For this review, take the finished solid that the model builds, in its own axes (mm). A direction names the side the tool comes from. Round coordinates to 2 decimals unless told otherwise and drop trailing zeros. Write each loop counter-clockwise with the first axis right and the second up, starting at its lowest first coordinate (ties: lowest second). Pieces come first, ordered by that corner, then holes. Notation, with made-up numbers: (-39, 57.5) -> (-18, 57.5) arc R25 cw to (-18, 69.5) -> close; hole circle Ø10 at (-17, -16). An arc over 180 degrees is marked (long way). Write each question's results on one line, items separated by ' | '. Start each with the question number.
Item 1: Clearance check with flat-ended pins moving along their axes: pin 1 (0.9 mm diameter, centred on y = 0, z = 1, fed in from +X) (3 decimals); pin 2 (4 mm diameter, centred on x = -9, y = -5, fed in from -Z). State where each tip first meets the part, or that it passes through.
Item 2: The part is to be moulded in two halves that separate along X. For faces 1 (the flat face through (25, -16, 2)), 2 (the flat face through (-16, -25, 2)), 3 (the flat face through (-6, 21.925, 2)), 4 (the flat face through (-25, 16, 2)), say which applies: +X half, -X half, draft (parallel to the pull), parting line (faces both ways), or undercut.
Item 3: Tool access review of faces 5 (the flat face through (-7.725, -23, 2)), 6 (the flat face through (6, 21.925, 2)), 7 (the flat face through (-23, 4.675, 2)), 8 (the flat face through (23, 7.725, 2)): name each direction out of +Z, -Z, +X, -X, +Y, -Y from which nothing blocks a thin tool from reaching the whole face with its end or side.
Item 4: To check wall thickness, follow line 1 along Y through (x, z) = (22, 0.6) (3 decimals); line 2 along X through (y, z) = (5.5, 1.5) (3 decimals). State the ranges of each line that lie inside material, in increasing order.
Item 5: Add section A-A (y = -5.5). State the section outline as (x, z) points (3 decimals), plus the area to 3 significant figures.
Autodesk Inventor part; units mm, degrees
ref_plane "YZ Plane" through (0, 0, 0) normal (1, 0, 0) x (0, 1, 0)
ref_plane "XZ Plane" through (0, 0, 0) normal (0, 1, 0) x (-1, 0, 0)
ref_plane "XY Plane" through (0, 0, 0) normal (0, 0, 1) x (1, 0, 0)
sketch "slots" plane through (0, 0, 0) normal (0, 0, 1) x (1, 0, 0)
  line L0 (61.2067, 31.1821) -> (64.2567, 31.1821)
  line L1 (64.2567, 31.1821) -> (64.2567, 28.1071)
  line L2 (64.2567, 28.1071) -> (61.2067, 28.1071)
  line L3 (61.2067, 28.1071) -> (61.2067, 31.1821)
  line L4 (68.9317, 33.8834) -> (68.9317, 26.9198) construction
  line L5 (67.4067, 31.1821) -> (70.4567, 31.1821)
  line L6 (70.4567, 31.1821) -> (70.4567, 28.1071)
  line L7 (70.4567, 28.1071) -> (67.4067, 28.1071)
  line L8 (67.4067, 28.1071) -> (67.4067, 31.1821)
  line L9 (73.6067, 31.1821) -> (76.6567, 31.1821)
  line L10 (76.6567, 31.1821) -> (76.6567, 28.1071)
  line L11 (76.6567, 28.1071) -> (73.6067, 28.1071)
  line L12 (73.6067, 28.1071) -> (73.6067, 31.1821)
  line L13 (68.9317, 28.1071) -> (68.9317, 27.1937) construction
  point P0 (68.8645, 30.3856)
  dimension "d2" = 3.05
  dimension "d3" = 3.075
  dimension "d4" = 3.15
  dimension "d5" = 3.15
sketch "Sketch1" plane through (0, 0, 0) normal (0, 0, 1) x (1, 0, 0)
  line L0 (-25, 25) -> (25, 25)
  line L1 (25, 25) -> (25, -25)
  line L2 (25, -25) -> (-25, -25)
  line L3 (-25, -25) -> (-25, 25)
  line L4 (0, 40.2669) -> (0, -57.9846) construction
  line L5 (-45.3823, 0) -> (61.3149, 0) construction
  line L6 (-7.725, 25) -> (-4.675, 25)
  line L7 (-4.675, 25) -> (-4.675, 21.925)
  line L8 (-4.675, 21.925) -> (-7.725, 21.925)
  line L9 (-7.725, 21.925) -> (-7.725, 25)
  line L10 (0, 27.7013) -> (0, 20.7377) construction
  line L11 (-1.525, 25) -> (1.525, 25)
  line L12 (1.525, 25) -> (1.525, 21.925)
  line L13 (1.525, 21.925) -> (-1.525, 21.925)
  line L14 (-1.525, 21.925) -> (-1.525, 25)
  line L15 (4.675, 25) -> (7.725, 25)
  line L16 (7.725, 25) -> (7.725, 21.925)
  line L17 (7.725, 21.925) -> (4.675, 21.925)
  line L18 (4.675, 21.925) -> (4.675, 25)
  line L19 (0, 21.925) -> (0, 21.0116) construction
  line L20 (-7.725, -21.925) -> (-4.675, -21.925)
  line L21 (-4.675, -21.925) -> (-4.675, -25)
  line L22 (-4.675, -25) -> (-7.725, -25)
  line L23 (-7.725, -25) -> (-7.725, -21.925)
  line L24 (0, -19.2237) -> (0, -26.1873) construction
  line L25 (-1.525, -21.925) -> (1.525, -21.925)
  line L26 (1.525, -21.925) -> (1.525, -25)
  line L27 (1.525, -25) -> (-1.525, -25)
  line L28 (-1.525, -25) -> (-1.525, -21.925)
  line L29 (4.675, -21.925) -> (7.725, -21.925)
  line L30 (7.725, -21.925) -> (7.725, -25)
  line L31 (7.725, -25) -> (4.675, -25)
  line L32 (4.675, -25) -> (4.675, -21.925)
  line L33 (0, -25) -> (0, -25.9134) construction
  line L34 (-25, -7.725) -> (-25, -4.675)
  line L35 (-25, -4.675) -> (-21.925, -4.675)
  line L36 (-21.925, -4.675) -> (-21.925, -7.725)
  line L37 (-21.925, -7.725) -> (-25, -7.725)
  line L38 (-27.7013, 0) -> (-20.7377, 0) construction
  line L39 (-25, -1.525) -> (-25, 1.525)
  line L40 (-25, 1.525) -> (-21.925, 1.525)
  line L41 (-21.925, 1.525) -> (-21.925, -1.525)
  line L42 (-21.925, -1.525) -> (-25, -1.525)
  line L43 (-25, 4.675) -> (-25, 7.725)
  line L44 (-25, 7.725) -> (-21.925, 7.725)
  line L45 (-21.925, 7.725) -> (-21.925, 4.675)
  line L46 (-21.925, 4.675) -> (-25, 4.675)
  line L47 (-21.925, 0) -> (-21.0116, 0) construction
  line L48 (21.925, -7.725) -> (21.925, -4.675)
  line L49 (21.925, -4.675) -> (25, -4.675)
  line L50 (25, -4.675) -> (25, -7.725)
  line L51 (25, -7.725) -> (21.925, -7.725)
  line L52 (19.2237, 0) -> (26.1873, 0) construction
  line L53 (21.925, -1.525) -> (21.925, 1.525)
  line L54 (21.925, 1.525) -> (25, 1.525)
  line L55 (25, 1.525) -> (25, -1.525)
  line L56 (25, -1.525) -> (21.925, -1.525)
  line L57 (21.925, 4.675) -> (21.925, 7.725)
  line L58 (21.925, 7.725) -> (25, 7.725)
  line L59 (25, 7.725) -> (25, 4.675)
  line L60 (25, 4.675) -> (21.925, 4.675)
  line L61 (25, 0) -> (25.9134, 0) construction
  point P0 (0, 0)
  point P1 (25, 0)
  point P2 (0, 25)
  dimension "d0" = 50
  dimension "d1" = 50
extrude "Extrusion1" add sketch "Sketch1" along normal blind 3.1 contours L0 L9 L8 L7 L14 L13 L12 L18 L17 L16 L1 L58 L57 L60 L54 L53 L56 L49 L48 L51 L2 L30 L29 L32 L26 L25 L28 L21 L20 L23 L3 L37 L36 L35 L42 L41 L40 L46 L45 L44
equation "\"d2\" = mat - kerf"
equation "\"d3\" = mat - 0.5 * kerf"
equation "\"d4\" = mat + kerf"
equation "\"d5\" = mat + kerf"
equation "\"d8\" = mat"
properties part number "base"
Responses:
1) pin 1: stops at x = 21.925 | pin 2: stops at z = 0
2) face 1: +X half | face 2: draft | face 3: undercut | face 4: -X half
3) face 5: +Z, -Z, -Y | face 6: +Z, -Z, +Y | face 7: +Z, -Z, -X | face 8: +Z, -Z, +X
4) line 1: y = -25 to -7.725, -4.675 to -1.525, 1.525 to 4.675, 7.725 to 25 | line 2: x = -21.925 to 21.925
5) outline: (-21.925, 0) -> (21.925, 0) -> (21.925, 3.1) -> (-21.925, 3.1) -> close | area: 136 mm^2
